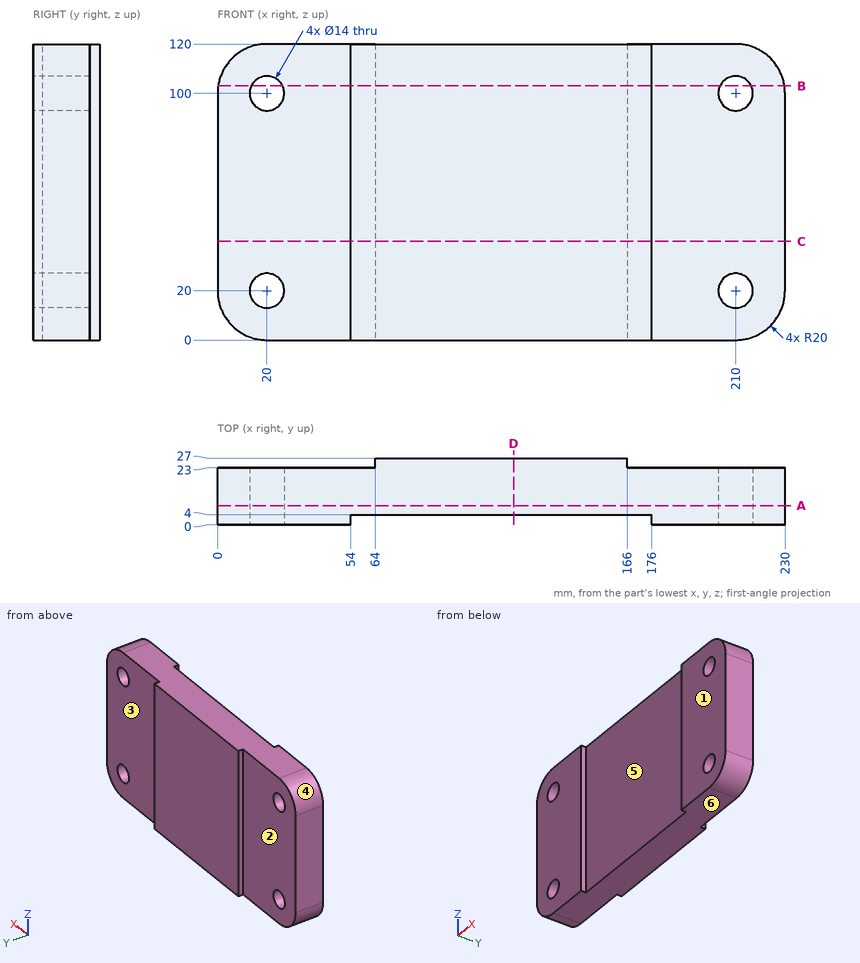
For this review, use the dimensioned drawing (mm, ordinates from the lowest corner) and the shaded views. A direction names the side the tool comes from. Coordinates: 2 decimals unless noted, no trailing zeros. Write each loop counter-clockwise with the first axis right and the second up, starting at its lowest first coordinate (ties: lowest second). Pieces come first, ordered by that corner, then holes. Notation, with made-up numbers: (53, 88) -> (67, 88) arc R21 cw to (67, 117) -> close; hole circle Ø5 at (-10.75, -25.75). An arc over 180 degrees is marked (long way). Put each result on its own line as item: value.
Q1. Clearance check with flat-ended pins moving along their axes: pin 1 Ø8 at (x, z) = (124, 23.5) entering from -Y; pin 2 Ø3 at (x, z) = (175, 102) entering from +Y; pin 3 Ø2 at (y, z) = (25.5, 69) entering from +X. State where each tip first meets the part, or that it passes through.
From the geometry:
pin 1: stops at y = 4
pin 2: stops at y = 23
pin 3: stops at x = 166
Q2. Take a section at A-A, the plane y = 7.75. State the section outline as (x, z) points, then the cut area to 3 significant figures.
From the geometry:
outline: (0, 20) arc R20 ccw to (20, 0) -> (210, 0) arc R20 ccw to (230, 20) -> (230, 100) arc R20 ccw to (210, 120) -> (20, 120) arc R20 ccw to (0, 100) -> close; hole circle Ø14 at (20, 20); hole circle Ø14 at (20, 100); hole circle Ø14 at (210, 20); hole circle Ø14 at (210, 100)
area: 26,600 mm2
Q3. The part is to be moulded in two halves that separate along X. For the marked faces 4, 5 and 6, say which applies: +X half, -X half, draft (parallel to the pull), parting line (faces both ways), or undercut.
From the geometry:
face 4: -X half
face 5: undercut
face 6: draft
Q4. Take a section at B-B, the plane z = 103. State the section outline as (x, y) points.
From the geometry:
outline: (0.23, 0) -> (13.68, 0) -> (13.68, 23) -> (0.23, 23) -> close; (26.32, 0) -> (54, 0) -> (54, 4) -> (176, 4) -> (176, 0) -> (203.68, 0) -> (203.68, 23) -> (166, 23) -> (166, 27) -> (64, 27) -> (64, 23) -> (26.32, 23) -> close; (216.32, 0) -> (229.77, 0) -> (229.77, 23) -> (216.32, 23) -> close
Q5. Wall thickness on L1, parallel to X at y = 12.75, z = 20; L2, parallel to X at y = 4.25, z = 98; L3, parallel to Y at x = 195.5, z = 69: over which ranges is each line inside the solid? List them lowest first.
From the geometry:
L1: x = 0 to 13, 27 to 203, 217 to 230
L2: x = 0 to 13.29, 26.71 to 203.29, 216.71 to 230
L3: y = 0 to 23
Q6. Tool access review of the marked faces 1, 2 and 3: name each direction out of +Z, -Z, +X, -X, +Y, -Y from which nothing blocks a thin tool from reaching the whole face with its end or side.
From the geometry:
face 1: +Z, -Z, +X, -X, -Y
face 2: +Z, -Z, -X, +Y
face 3: +Z, -Z, +X, +Y
Q7. Take a section at D-D, the plane x = 120. State the section outline as (y, z) points, then the cut area to 3 significant figures.
From the geometry:
outline: (4, 0) -> (27, 0) -> (27, 120) -> (4, 120) -> close
area: 2,760 mm2
Q8. Take a section at C-C, the plane z = 40. State the section outline as (x, y) points, then the cut area to 3 significant figures.
From the geometry:
outline: (0, 0) -> (54, 0) -> (54, 4) -> (176, 4) -> (176, 0) -> (230, 0) -> (230, 23) -> (166, 23) -> (166, 27) -> (64, 27) -> (64, 23) -> (0, 23) -> close
area: 5,210 mm2
